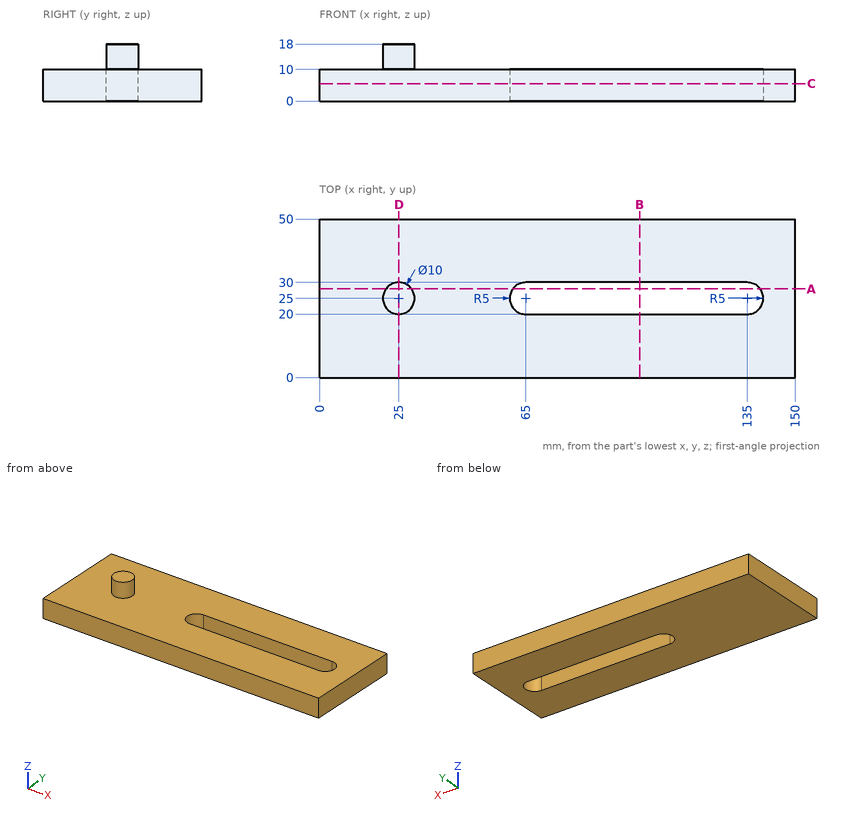
Print and shaded views of the part. All mm, measured from the part's lowest x, y and z. Give positions to 0.01 mm unless a question says otherwise; leave off trailing zeros. Write each loop counter-clockwise with the first axis right and the second up, starting at its lowest first coordinate (ties: lowest second). Pieces come first, ordered by that corner, then holes. Notation, with made-up numbers: (-13, -4.75) - (-7, -4.75) arc R20 ccw to (-7, 11.25) - close; hole circle Ø4 at (63, 42). An arc over 180 degrees is marked (long way). Put each result on its own line as item: value.
(1) Saw through at A-A (y = 28). List the corners of the cut face in (x, z), then the cut area to 3 significant figures.
Working result:
outline: (0, 0) - (61, 0) - (61, 10) - (29, 10) - (29, 18) - (21, 18) - (21, 10) - (0, 10) - close; (139, 0) - (150, 0) - (150, 10) - (139, 10) - close
area: 784 mm^2
(2) Saw through at C-C (z = 5.5). List the corners of the cut face in (x, y).
Working result:
outline: (0, 0) - (150, 0) - (150, 50) - (0, 50) - close; hole (65, 20) - (135, 20) arc R5 ccw to (135, 30) - (65, 30) arc R5 ccw to start
(3) Wall check: L1, parallel to Y at x = 96, z = 9.75; L2, parallel to Z at x = 20, y = 33.5; L3, parallel to X at y = 29.5, z = 4. Give the ranges that are in metal, low to high.
Working result:
L1: 0 to 20, 30 to 50
L2: 0 to 10
L3: 0 to 62.82, 137.18 to 150
(4) Saw through at B-B (x = 101). List the corners of the cut face in (y, z), then the cut area to 3 significant figures.
Working result:
outline: (0, 0) - (20, 0) - (20, 10) - (0, 10) - close; (30, 0) - (50, 0) - (50, 10) - (30, 10) - close
area: 400 mm^2
(5) Drop flat-ended pins along their axis: pin 1 Ø3 at (x, y) = (76.5, 35.5) entering from -Z; pin 2 Ø12 at (x, y) = (21.5, 14) entering from +Z. Give the stop position or say it passes through.
Working result:
pin 1: z = 0
pin 2: z = 10
(6) Saw through at D-D (x = 25). List the corners of the cut face in (y, z).
Working result:
outline: (0, 0) - (50, 0) - (50, 10) - (30, 10) - (30, 18) - (20, 18) - (20, 10) - (0, 10) - close
